Autodesk Inventor part; units mm, degrees
ref_plane "YZ Plane" through (0, 0, 0) normal (1, 0, 0) x (0, 1, 0)
ref_plane "XZ Plane" through (0, 0, 0) normal (0, 1, 0) x (-1, 0, 0)
ref_plane "XY Plane" through (0, 0, 0) normal (0, 0, 1) x (1, 0, 0)
sketch "Эскиз6" plane through (0, 0, 0) normal (1, 0, 0) x (0, 1, 0)
  circle A0 centre (0, 0) radius 9.5
  circle A1 centre (0, 0) radius 5
  dimension "d13" = 19
  dimension "d14" = 10
extrude "Выдавливание5" add sketch "Эскиз6" along normal blind 5
sketch "Эскиз7" plane through (5, 0, 0) normal (1, 0, 0) x (0, 0, -1)
  circle A0 centre (0, 0) radius 6
  circle A1 centre (0, 0) radius 8.5
  dimension "d17" = 12
  dimension "d18" = 17
extrude "Выдавливание6" cut sketch "Эскиз7" against normal blind 0.5
sketch "Эскиз8" plane through (0, 0, 0) normal (-1, 0, 0) x (0, 0, 1)
  circle A0 centre (0, 0) radius 6
  circle A1 centre (0, 0) radius 8.4142
extrude "Выдавливание7" cut sketch "Эскиз8" against normal blind 0.5
properties part number "подшипник для ведущих шестеренок" material "Титан"
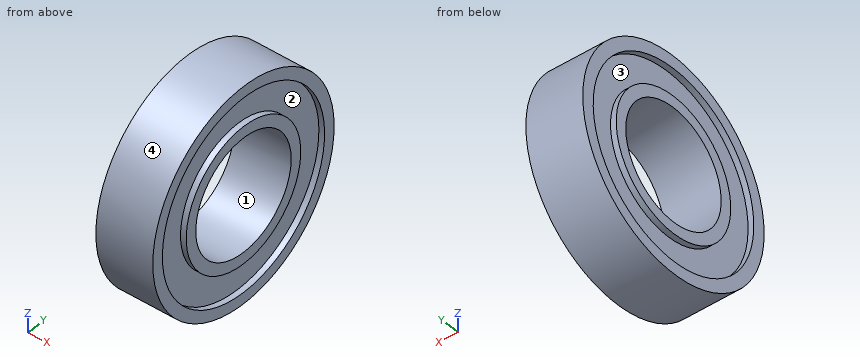
Could you check a few things on this model? Use its own coordinates, in mm. Face numbers are marked on the shaded views. A direction names the side the tool comes from. Give positions to 0.01 mm unless a question says otherwise; leave off trailing zeros. Loops run counter-clockwise (first coordinate to the right, second up) from the corner with the lowest first, then second, coordinate; pieces in that order, holes last. Notation, with made-up numbers: (71.5, 79) - (115.5, 79) arc R14 cw to (115.5, 106) - close; hole circle Ø6 at (29, 37). An arc over 180 degrees is marked (long way). Answer in a Markdown table with one row per item. Add a question column.
Q1. We'd pull the mould along Z, two halves only. Please class the marked faces 3 and 4: +Z half, -Z half, draft (parallel to the pull), parting line (faces both ways), or undercut.
Q2. If we section it at D-D (y = -6.5): List the corners of the cut face in (x, z) for me.
Q3. If we section it at C-C (x = 2.85): List the corners of the cut face in (y, z) for me.
Q4. Which directions (+Z, -Z, +X, -X, +Y, -Y) give clear straight access to the entire face, cutting with the end or side of a thin tool? Please do the marked faces 1 and 2.
Q5. For pin 1 (1 mm diameter, centred on x = 3, y = -2.5, fed in from -Z); pin 2 (1.5 mm diameter, centred on x = 2.5, z = 4.5, fed in from -Y), each with a flat end and sliding along its axis, tell me the tip position at first contact or that it passes through.
Q6. If we section it at A-A (z = 0): List the corners of the cut face in (x, y) for me, plus the area to 3 significant figures.
Q7. Please list where these lines run through material, in increasing order: L1, parallel to Z at x = 1.55, y = 0; L2, parallel to X at y = -6.25, z = -4.5; L3, parallel to Y at x = 3.25, z = 0.25. Write a range as from..to.
The answers:
| question | item | result |
|---|---|---|
| 1 | face 3 | undercut |
| 1 | face 4 | parting line |
| 2 | outline | (0, -6.93) - (5, -6.93) - (5, -5.48) - (4.5, -5.48) - (4.5, 5.48) - (5, 5.48) - (5, 6.93) - (0, 6.93) - (0, 5.34) - (0.5, 5.34) - (0.5, -5.34) - (0, -5.34) - close |
| 3 | outline | circle Ø19 at (0, 0); hole circle Ø10 at (0, 0) |
| 4 | face 1 | +X, -X |
| 4 | face 2 | +X |
| 5 | pin 1 | stops at z = -9.29 |
| 5 | pin 2 | stops at y = -8.73 |
| 6 | outline | (0, -9.5) - (5, -9.5) - (5, -8.5) - (4.5, -8.5) - (4.5, -6) - (5, -6) - (5, -5) - (0, -5) - (0, -6) - (0.5, -6) - (0.5, -8.41) - (0, -8.41) - close; (0, 5) - (5, 5) - (5, 6) - (4.5, 6) - (4.5, 8.5) - (5, 8.5) - (5, 9.5) - (0, 9.5) - (0, 8.41) - (0.5, 8.41) - (0.5, 6) - (0, 6) - close |
| 6 | area | 40.1 mm^2 |
| 7 | L1 | z = -9.5..-5, 5..9.5 |
| 7 | L2 | x = 0.5..4.5 |
| 7 | L3 | y = -9.5..-4.99, 4.99..9.5 |
